Autodesk Inventor part; units mm, degrees
ref_plane "YZ Plane" through (0, 0, 0) normal (1, 0, 0) x (0, 1, 0)
ref_plane "XZ Plane" through (0, 0, 0) normal (0, 1, 0) x (-1, 0, 0)
ref_plane "XY Plane" through (0, 0, 0) normal (0, 0, 1) x (1, 0, 0)
sketch "Sketch1" plane through (0, 0, 0) normal (0, 0, 1) x (1, 0, 0)
  line L0 (-279.4, 38.1) -> (279.4, 38.1)
  line L1 (279.4, 38.1) -> (279.4, -38.1)
  line L2 (279.4, -38.1) -> (-279.4, -38.1)
  line L3 (-279.4, -38.1) -> (-279.4, 38.1)
  line L4 (0, 0) -> (0, 412.8984) construction
  line L5 (0, 0) -> (748.8943, 0) construction
  dimension "d0" = 558.8
  dimension "d1" = 76.2
  dimension "d2" = 38.1
  dimension "d4" = 279.4
extrude "Extrusion1" add sketch "Sketch1" along normal mid plane 1143
sketch "Sketch2" plane through (-279.4, 38.1, 571.5) normal (0, 1, 0) x (1, 0, 0)
  line L0 (558.8, 0) -> (558.8, 1143)
  line L1 (0, 1143) -> (0, 0)
  line L2 (558.8, 1143) -> (0, 1143)
  line L3 (0, 1143) -> (0, 1066.8)
  line L4 (0, 1066.8) -> (558.8, 1066.8)
  line L5 (558.8, 1066.8) -> (558.8, 1143)
  point P0 (279.4, 571.5)
  dimension "d7" = 76.2
extrude "Extrusion2" add sketch "Sketch2" along normal blind 762
mirror "Mirror1" about plane through (0, 0, 0) normal (0, 0, 1) of "Extrusion2"
sketch "Sketch3" plane through (-279.4, 38.1, -495.3) normal (0, 1, 0) x (1, 0, 0)
  circle A0 centre (279.4, -495.3) radius 101.6
  circle A1 centre (279.4, -292.1) radius 25.4
  line L0 (558.8, -990.6) -> (558.8, 0)
  circle A2 centre (423.0841, -351.6159) radius 25.4
  circle A3 centre (482.6, -495.3) radius 25.4
  circle A4 centre (423.0841, -638.9841) radius 25.4
  circle A5 centre (279.4, -698.5) radius 25.4
  dimension "d10" = 203.2
  dimension "d11" = 50.8
  dimension "d12" = 203.2
  dimension "d13" = 279.4
  dimension "d16" = 180
extrude "Extrusion3" cut sketch "Sketch3" against normal through all
sketch "Sketch4" plane through (0, 0, -571.5) normal (0, 0, -1) x (-1, 0, 0)
  line L0 (-314.4934, 723.9) -> (334.7896, 723.9) construction
  line L1 (279.4, 800.1) -> (-279.4, 800.1) construction
  arc A0 (-101.6, 723.9) -> (101.6, 723.9) centre (0, 723.9) ccw
  line L2 (279.4, -38.1) -> (279.4, 800.1)
  line L3 (-279.4, 800.1) -> (279.4, 800.1)
  line L4 (101.6, 723.9) -> (101.6, 800.1)
  line L5 (-101.6, 723.9) -> (-101.6, 800.1)
  circle A1 centre (-203.2, 723.9) radius 25.4
  circle A2 centre (-143.6841, 580.2159) radius 25.4
  circle A3 centre (0, 520.7) radius 25.4
  circle A4 centre (143.6841, 580.2159) radius 25.4
  circle A5 centre (203.2, 723.9) radius 25.4
  point P0 (0, 0)
  dimension "d20" = 76.2
  dimension "d21" = 203.2
  dimension "d22" = 279.4
  dimension "d23" = 50.8
  dimension "d24" = 203.2
  dimension "d27" = 180
extrude "Extrusion4" cut sketch "Sketch4" against normal through all
fillet "Fillet1" radius 50.8 10 edges at (101.6, 800.1, -533.4) (-101.6, 800.1, -533.4) (-101.6, 800.1, 533.4) (101.6, 800.1, 533.4) (279.4, 800.1, 533.4) (-279.4, 800.1, 533.4) (279.4, 800.1, -533.4) (-279.4, 800.1, -533.4) (0, -38.1, -571.5) (0, -38.1, 571.5)
properties part number "Down_Part_Robot"
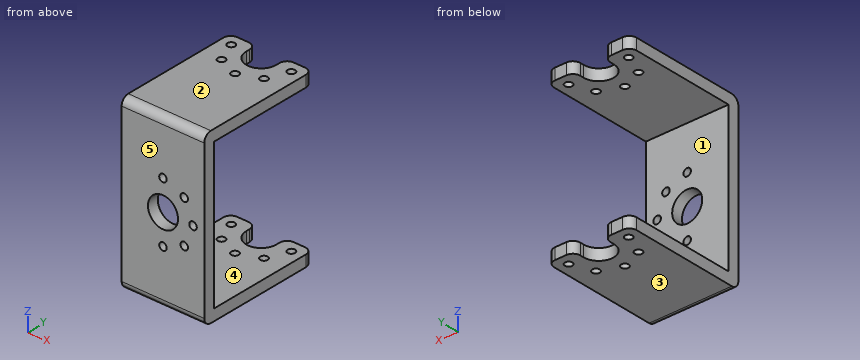
Design review of the part built by this model. Coordinates are the model's own, in mm. Face numbers are marked on the shaded views. A direction names the side the tool comes from. Give positions to 0.01 mm unless a question says otherwise; leave off trailing zeros. Order: outer loops, then holes, each group sorted by start corner. A loop starts at its lowest first (then second) coordinate and runs counter-clockwise, first axis right, second up. Notation, with made-up numbers: (79.25, -29) - (102.25, -29) arc R14 ccw to (102.25, -13) - close; hole circle Ø2 at (-9, 7.5). An arc over 180 degrees is marked (long way). Use CSV: the item, a comma, the result in double quotes. Start each with the question number.
Q1. For P1, Ø1, axis at x = 153, z = -93, coming from the +Y side, flat-tipped, find the tip position at first contact; note if it passes through.
Q2. Take a section at C-C (x = 0). Count the separate pieces of the cut face and the enclosed holes in it, and give its area (3 significant figures).
Q3. Draft analysis for pull direction Z (two halves, no side actions). For the marked faces 3, 4 and 5, state which applies: pulls with the +Z half, pulls with the -Z half, needs draft (parallel to the pull), parting line crosses it, or undercut.
Q4. Machinability: for the marked faces 1 and 2, which of the approach directions +Z, -Z, +X, -X, +Y, -Y give a long, thin tool a straight path to every point of the face, cutting with its end or side? Answer none if there is none.
Q5. Take a section at D-D (x = -203.2). State the section outline as (y, z) points.
Q6. Take a section at B-B (y = 312). State the section outline as (x, z) points, and give its area (3 significant figures).
Q7. Take a section at A-A (z = 0). State the section outline as (x, y) points, and give its area (3 significant figures).
Q8. For line 1 (Y direction, x = 0, z = 520); line 2 (Z direction, x = -210, y = 200.5); line 3 (Y direction, x = 203.2, z = 518), list the stretches that pass through material, from the lowest coordinate up.
Calculated:
1,P1,"stops at y = 38.1"
2,separate pieces,"6"
2,enclosed holes,"0"
2,area,"144,000 mm²"
3,face 3,"pulls with the -Z half"
3,face 4,"undercut"
3,face 5,"needs draft"
4,face 1,"+X, -X, +Y"
4,face 2,"+Z, +X, -X, +Y, -Y"
5,outline,"(-38.1, -520.7) arc R50.8 ccw to (12.7, -571.5) - (698.5, -571.5) - (698.5, -495.3) - (38.1, -495.3) - (38.1, 495.3) - (698.5, 495.3) - (698.5, 571.5) - (12.7, 571.5) arc R50.8 ccw to (-38.1, 520.7) - close; (749.3, -571.5) - (800.1, -571.5) - (800.1, -495.3) - (749.3, -495.3) - close; (749.3, 495.3) - (800.1, 495.3) - (800.1, 571.5) - (749.3, 571.5) - close"
6,outline,"(-279.4, -571.5) - (279.4, -571.5) - (279.4, -495.3) - (-279.4, -495.3) - close; (-279.4, 495.3) - (279.4, 495.3) - (279.4, 571.5) - (-279.4, 571.5) - close"
6,area,"85,200 mm²"
7,outline,"(-279.4, -38.1) - (-101.6, -38.1) - (-101.6, 38.1) - (-279.4, 38.1) - close; (101.6, -38.1) - (177.8, -38.1) - (177.8, 38.1) - (101.6, 38.1) - close; (228.6, -38.1) - (279.4, -38.1) - (279.4, 38.1) - (228.6, 38.1) - close"
7,area,"23,200 mm²"
8,line 1,"y = -38.1 to 495.3, 546.1 to 622.3"
8,line 2,"z = -571.5 to -495.3, 495.3 to 571.5"
8,line 3,"y = -38.1 to 698.5, 749.3 to 800.1"
